Autodesk Inventor part; units mm, degrees
ref_plane "YZ Plane" through (0, 0, 0) normal (1, 0, 0) x (0, 1, 0)
ref_plane "XZ Plane" through (0, 0, 0) normal (0, 1, 0) x (-1, 0, 0)
ref_plane "XY Plane" through (0, 0, 0) normal (0, 0, 1) x (1, 0, 0)
sketch "스케치1" plane through (0, 0, 0) normal (0, 0, 1) x (1, 0, 0)
  line L0 (0, 0) -> (-14, 0)
  line L1 (-14, 6) -> (-14, 18)
  line L2 (-14, 18) -> (0, 18)
  line L3 (0, 18) -> (0, 0)
  line L4 (-14, 0) -> (-30, 0)
  line L5 (-30, 0) -> (-30, 12)
  line L6 (-30, 12) -> (-24, 12)
  line L7 (-24, 12) -> (-24, 6)
  line L8 (-24, 6) -> (-14, 6)
  line L9 (-7, 13) -> (-7, 5) construction
  line L10 (-10, 13) -> (-10, 5)
  line L11 (-4, 5) -> (-4, 13)
  arc A0 (-4, 13) -> (-10, 13) centre (-7, 13) ccw
  arc A1 (-10, 5) -> (-4, 5) centre (-7, 5) ccw
  point P0 (-7, 9)
  dimension "d0" = 14
  dimension "d3" = 12
  dimension "d4" = 6
  dimension "d5" = 10
  dimension "d6" = 30
  dimension "d7" = 6
  dimension "d8" = 8
  dimension "d9" = 5
  dimension "d10" = 7
  dimension "d11" = 18
extrude "돌출1" add sketch "스케치1" along normal mid plane 15
chamfer "모따기1" distance 3 angle 45 3 edges at (-14, 18, 0) (0, 18, 0) (0, 0, 0)
sketch "스케치2" plane through (0, 0, 0) normal (0, 0, 1) x (1, 0, 0)
  line L0 (-17, 20.9368) -> (7.8455, 20.9368)
  line L1 (7.8455, 20.9368) -> (7.8455, -4.4634)
  line L2 (7.8455, -4.4634) -> (-17, -4.4634)
  line L3 (-17, -4.4634) -> (-17, 20.9368)
  line L4 (0, 15) -> (0, 3)
  point P0 (0, 0)
  dimension "d17" = 17
extrude "돌출2" cut sketch "스케치2" along normal mid plane 8
properties part number "14-2"
Build history of the part. All positions in model axes, mm. A direction names the side the tool comes from. Give positions to 0.01 mm unless a question says otherwise; leave off trailing zeros. Loops run counter-clockwise (first coordinate to the right, second up) from the corner with the lowest first, then second, coordinate; pieces in that order, holes last.
Item 1: Flat gauge pins, fed straight in: pin 1 (3 mm diameter, centred on y = 4, z = 1, fed in from +X); pin 2 (5 mm diameter, centred on x = -28.5, z = -3, fed in from +Y). Where does each tip first touch, or does it go through?
Answers follow:
pin 1: stops at x = -17
pin 2: stops at y = 12
Item 2: Slice it at D-D, the plane z = -2. List the corners of the cut face in (x, y), and give its area (3 significant figures).
Answers follow:
outline: (-30, 0) - (-17, 0) - (-17, 6) - (-24, 6) - (-24, 12) - (-30, 12) - close
area: 114 mm2
Item 3: Which spindle directions (+Z, -Z, +X, -X, +Y, -Y) get a long thin tool onto all of the face, cutting with end or side? Do faces 1 (the face through (-7, 16, 6)), 2 (the face through (-24, 9, 0)), 3 (the face through (-19, 0, 0)), 4 (the face through (-11, 9, 4)). Say none if no direction does.
Answers follow:
face 1: +Z, -Z
face 2: +Z, -Z, +Y
face 3: +Z, -Z, +X, -X, -Y
face 4: +X, +Y, -Y
Item 4: Slice it at A-A, the plane x = -7. List the corners of the cut face in (y, z).
Answers follow:
outline: (0, -7.5) - (2, -7.5) - (2, -4) - (0, -4) - close; (0, 4) - (2, 4) - (2, 7.5) - (0, 7.5) - close; (16, -7.5) - (18, -7.5) - (18, -4) - (16, -4) - close; (16, 4) - (18, 4) - (18, 7.5) - (16, 7.5) - close
Item 5: Drill centre lines: line 1 (X direction, y = 11.25, z = 4.75); line 2 (Z direction, x = -13.75, y = 12); line 3 (X direction, y = 9.25, z = 1.75). Where is each one in solid material? Low to high.
Answers follow:
line 1: x = -30 to -24, -14 to -10, -4 to 0
line 2: z = -7.5 to -4, 4 to 7.5
line 3: x = -30 to -24
Item 6: Slice it at C-C, the plane y = 2.5. List the corners of the cut face in (x, z), and give its area (3 significant figures).
Answers follow:
outline: (-30, -7.5) - (-8.66, -7.5) - (-8.66, -4) - (-17, -4) - (-17, 4) - (-8.66, 4) - (-8.66, 7.5) - (-30, 7.5) - close; (-5.34, -7.5) - (-0.5, -7.5) - (-0.5, -4) - (-5.34, -4) - close; (-5.34, 4) - (-0.5, 4) - (-0.5, 7.5) - (-5.34, 7.5) - close
area: 287 mm2
Item 7: Pull direction Z, two halves, no side cores. Call faces 5 (the face through (-7, 16, -6)), 6 (the face through (-15, 5, -7.5)), 7 (the face through (-11, 9, -4)): released by +Z, released by -Z, zero draft, split by the parting line, or undercut.
Answers follow:
face 5: zero draft
face 6: released by -Z
face 7: undercut
Item 8: Slice it at B-B, the plane y = 10.5. List the corners of the cut face in (x, z), and give its area (3 significant figures).
Answers follow:
outline: (-30, -7.5) - (-24, -7.5) - (-24, 7.5) - (-30, 7.5) - close; (-14, -7.5) - (-10, -7.5) - (-10, -4) - (-14, -4) - close; (-14, 4) - (-10, 4) - (-10, 7.5) - (-14, 7.5) - close; (-4, -7.5) - (0, -7.5) - (0, -4) - (-4, -4) - close; (-4, 4) - (0, 4) - (0, 7.5) - (-4, 7.5) - close
area: 146 mm2
